Part model, mm, in its own coordinate system. Round coordinates to 2 decimals unless told otherwise and drop trailing zeros. Loops run counter-clockwise (first coordinate to the right, second up) from the corner with the lowest first, then second, coordinate; pieces in that order, holes last. Notation, with made-up numbers: (69.25, 46) -> (101.25, 46) arc R18 cw to (101.25, 55) -> close; hole circle Ø3 at (-14.5, -23.75). An arc over 180 degrees is marked (long way). Use a Markdown table: item, result. Add a question column.
Item 1: Two-plate mould, pull along Z, no slides. Class faces 1 (the face through (1.5, 1.5, 0)), 2 (the face through (1, 1, -5.5)), 3 (the face through (0.41, 1.53, -3.15)), 4 (the face through (0, 1, 2)): pulls with the +Z half, pulls with the -Z half, needs draft (parallel to the pull), parting line crosses it, or undercut.
Item 2: Cut at D-D, the plane x = 1.1. List the corners of the cut face in (y, z) (3 decimals).
Item 3: Cut at B-B, the plane y = 1.5. List the corners of the cut face in (x, z).
Item 4: Cut at C-C, the plane x = 0.2. List the corners of the cut face in (y, z), plus the area to 3 significant figures.
Item 5: Probe line 1 (Y direction, x = 0.3, z = -3.75); line 2 (Y direction, x = 1.2, z = -3); line 3 (X direction, y = 0.6, z = -2.75). List the from-to ranges inside material, lowest first. Write a range as [from, to].
Item 6: Flat gauge pins, fed straight in: pin 1 (1.5 mm diameter, centred on x = 1.5, y = 2.5, fed in from +Z); pin 2 (1.5 mm diameter, centred on y = 2.5, z = 0, fed in from -X). Where does each tip first touch, or does it go through?
Item 7: Cut at A-A, the plane z = -3.75. List the corners of the cut face in (x, y), plus the area to 3 significant figures.
Autodesk Inventor part; units mm, degrees
ref_plane "YZ Plane" through (0, 0, 0) normal (1, 0, 0) x (0, 1, 0)
ref_plane "XZ Plane" through (0, 0, 0) normal (0, 1, 0) x (-1, 0, 0)
ref_plane "XY Plane" through (0, 0, 0) normal (0, 0, 1) x (1, 0, 0)
sketch "Sketch1" plane through (0, 0, 0) normal (0, 1, 0) x (-1, 0, 0)
  arc A0 (0, 1.5) -> (0, -1.5) centre (0, 0) ccw
  line L0 (0, 1.5) -> (0, 2.5)
  arc A1 (0, 2.5) -> (0, -2.5) centre (0, 0) ccw
  line L1 (0, -1.5) -> (0, -2.5)
  line L2 (0, -2.5) -> (-1.5, -2.5)
  line L3 (-1.5, -2.5) -> (-1.5, -5.5)
  line L4 (-1.5, -5.5) -> (0, -5.5)
  line L5 (0, -5.5) -> (0, -2.5)
  line L6 (-1.5, -2.5) -> (-1.5, -2)
  dimension "d0" = 1.5
  dimension "d1" = 1
  dimension "d2" = 1.5
  dimension "d3" = 3
extrude "Extrusion1" add sketch "Sketch1" along normal blind 3
sketch "Sketch2" plane through (1.5, 0, -2) normal (1, 0, 0) x (0, 0, -1)
  line L0 (0, 3) -> (3.5, 3)
  line L1 (1.75, 3) -> (1.75, 0) construction
  line L2 (3.5, 0) -> (3.5, 3)
  line L3 (3.5, 1.5) -> (1.75, 1.5) construction
  circle A0 centre (1.75, 1.5) radius 0.6
  point P0 (-2, 0)
  dimension "d6" = 1.2
extrude "Extrusion2" cut sketch "Sketch2" against normal blind 3
chamfer "Chamfer1" distance 0.7 angle 45 1 edges at (1.5, 1.5, -3.15)
properties part number "miniWiresHolder"
A:
| question | item | result |
|---|---|---|
| 1 | face 1 | undercut |
| 1 | face 2 | pulls with the -Z half |
| 1 | face 3 | undercut |
| 1 | face 4 | needs draft |
| 2 | outline | (0, -5.5) -> (3, -5.5) -> (3, -1.02) -> (0, -1.02) -> close; (0, 1.02) -> (3, 1.02) -> (3, 2.245) -> (0, 2.245) -> close; hole circle Ø1.8 at (1.5, -3.75) |
| 3 | outline | (0, -5.5) -> (1.5, -5.5) -> (1.5, -5.05) -> (0.8, -4.35) -> (0, -4.35) -> close; (0, -3.15) -> (0.8, -3.15) -> (1.5, -2.45) -> (1.5, -2) arc R2.5 ccw to (0, 2.5) -> (0, 1.5) arc R1.5 cw to (0, -1.5) -> close |
| 4 | outline | (0, -5.5) -> (3, -5.5) -> (3, -1.49) -> (0, -1.49) -> close; (0, 1.49) -> (3, 1.49) -> (3, 2.49) -> (0, 2.49) -> close; hole circle Ø1.2 at (1.5, -3.75) |
| 4 | area | 13.9 mm^2 |
| 5 | line 1 | y = [0, 0.9], [2.1, 3] |
| 5 | line 2 | y = [0, 0.84], [2.16, 3] |
| 5 | line 3 | x = [0, 1.5] |
| 6 | pin 1 | stops at z = 2.38 |
| 6 | pin 2 | stops at x = 1.3 |
| 7 | outline | (0, 0) -> (1.5, 0) -> (1.5, 0.2) -> (0.8, 0.9) -> (0, 0.9) -> close; (0, 2.1) -> (0.8, 2.1) -> (1.5, 2.8) -> (1.5, 3) -> (0, 3) -> close |
| 7 | area | 2.21 mm^2 |
